Geometry check sheet. Reference: the model listing, model coordinates, mm. Face numbers are marked on the shaded views. Give positions to 0.01 mm unless a question says otherwise; leave off trailing zeros. Write each loop counter-clockwise with the first axis right and the second up, starting at its lowest first coordinate (ties: lowest second). Pieces come first, ordered by that corner, then holes. Notation, with made-up numbers: (12.5, 82) -> (37.5, 82) arc R14 ccw to (37.5, 91) -> close; hole circle Ø10 at (83.5, 85.25). An arc over 180 degrees is marked (long way). One line per item, written item: value.
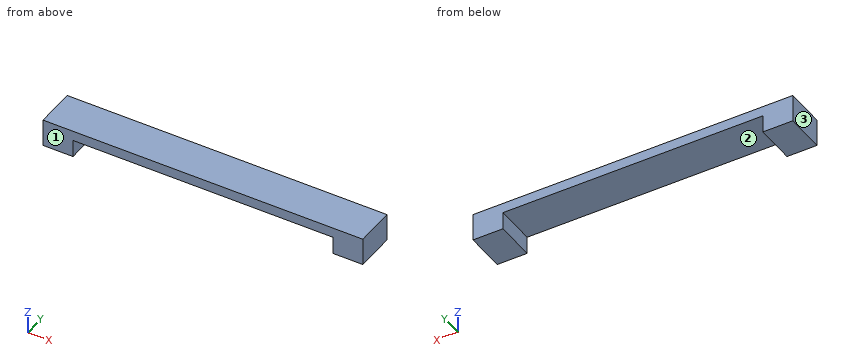
from build123d import *

# Parameters (mm, degrees)
BOX517_W     = 128
BOX517_H     = 16
BOX517_DEPTH = 4
BOX518_W     = 12
BOX518_H     = 16
BOX518_DEPTH = 11
BOX519_W     = 12
BOX519_H     = 16
BOX519_DEPTH = 11


with BuildPart() as box517:
    # Box517 → Box517 (new body)
    with BuildSketch(Plane(origin=(-98, -27, 47), x_dir=(1, 0, 0), z_dir=(0, 0, 1))):
        with Locations((64, 8)):
            Rectangle(BOX517_W, BOX517_H)
    extrude(amount=BOX517_DEPTH)


with BuildPart() as box518:
    # Box518 → Box518 (new body)
    with BuildSketch(Plane(origin=(-98, -27, 40), x_dir=(1, 0, 0), z_dir=(0, 0, 1))):
        with Locations((6, 8)):
            Rectangle(BOX518_W, BOX518_H)
    extrude(amount=BOX518_DEPTH)


with BuildPart() as fusion400:
    # Box519 → Box519 (new body)
    with BuildSketch(Plane(origin=(18, -27, 40), x_dir=(1, 0, 0), z_dir=(0, 0, 1))):
        with Locations((6, 8)):
            Rectangle(BOX519_W, BOX519_H)
    extrude(amount=BOX519_DEPTH)

    # Fusion400: union Box517, Box518
    add(box517.part)
    add(box518.part)


with BuildPart() as fusion400_1:
    # Fusion400 placement: moved
    add(fusion400.part.moved(Location((0, -29, 0))))


solid = fusion400_1.part
1) Sectioned sample at A-A on z = 41.25. Record the cut outline in (x, y), plus the area to 3 significant figures.
Verdict:
outline: (-98, -56) -> (-86, -56) -> (-86, -40) -> (-98, -40) -> close; (18, -56) -> (30, -56) -> (30, -40) -> (18, -40) -> close
area: 384 mm^2
2) Scan lines: probe 1 along X at (y, z) = (-46.5, 46.75); probe 2 along Z at (x, y) = (-1.5, -54.25). Record each from-to range of solid material in increasing order.
Verdict:
probe 1: -98 to -86, 18 to 30
probe 2: 47 to 51
3) Sectioned sample at B-B on y = -49. Record the cut outline in (x, z), plus the area to 3 significant figures.
Verdict:
outline: (-98, 40) -> (-86, 40) -> (-86, 47) -> (18, 47) -> (18, 40) -> (30, 40) -> (30, 51) -> (-98, 51) -> close
area: 680 mm^2
4) Depth check by flat-ended pin: pin 1 Ø8 at (x, y) = (-26.5, -46) entering from -Z. Enter the tip coordinate at first touch or a pass-through.
Verdict:
pin 1: z = 47
5) Sectioned sample at C-C on x = -67. Record the cut outline in (y, z), plus the area to 3 significant figures.
Verdict:
outline: (-56, 47) -> (-40, 47) -> (-40, 51) -> (-56, 51) -> close
area: 64.0 mm^2
6) Mould release check, pull along X, two halves, no side actions. Record for the marked faces 1, 2 and 3: released by +X, released by -X, zero draft, split by the parting line, or undercut.
Verdict:
face 1: zero draft
face 2: undercut
face 3: released by -X
